from build123d import *

# Parameters (mm, degrees)
EXTRUDE_THIN1_DEPTH = 492.125
FILLET1_R           = 1.016


with BuildPart() as part:
    # Sketch1 → Extrude-Thin1 (new body)
    with BuildSketch(Plane.XY):
        with BuildLine():
            Line((0, 6.35), (0, 0))
            Line((0, 0), (-6.35, 0))
            Line((-6.35, 0), (-6.35, 3.96875))
            ThreePointArc((-6.35, 3.96875), (-14.128687, 6.629724), (-18.647706, 13.497563))
            ThreePointArc((-18.647706, 13.497563), (-20.900169, 25.701402), (-21.43125, 38.1))
            Line((-21.43125, 38.1), (-23.8125, 38.1))
            Line((-23.8125, 38.1), (-23.8125, 49.2125))
            Line((-23.8125, 49.2125), (-17.4625, 48.879711))
            Line((-17.4625, 48.879711), (-17.515673, 47.865103))
            Line((-17.515673, 47.865103), (-22.7965, 48.141859))
            Line((-22.7965, 48.141859), (-22.7965, 39.116))
            Line((-22.7965, 39.116), (-20.381189, 39.116))
            ThreePointArc((-20.381189, 39.116), (-19.947758, 26.334511), (-17.66389, 13.751258))
            ThreePointArc((-17.66389, 13.751258), (-13.09767, 7.130154), (-5.334, 5.029008))
            Line((-5.334, 5.029008), (-5.334, 1.016))
            Line((-5.334, 1.016), (-1.016, 1.016))
            Line((-1.016, 1.016), (-1.016, 6.35))
            Line((-1.016, 6.35), (0, 6.35))
        make_face()
    extrude(amount=-EXTRUDE_THIN1_DEPTH)

    # Fillet1
    fillet1_edges = [part.edges().sort_by_distance(p)[0] for p in [
        (-20.381189, 39.116, -246.0625),
        (-5.334, 5.029008, -246.0625),
        (0, 0, -246.0625),
        (-6.35, 0, -246.0625),
        (-23.8125, 38.1, -246.0625),
        (-23.8125, 49.2125, -246.0625),
    ]]
    fillet(fillet1_edges, radius=FILLET1_R)


solid = part.part
CAD build for the part. Positions are in the model's coordinates, mm. Coordinates: 2 decimals unless noted, no trailing zeros. Order: outer loops, then holes, each group sorted by start corner. A loop starts at its lowest first (then second) coordinate and runs counter-clockwise, first axis right, second up.
Item 1: Two-plate mould, pull along X, no slides. Class faces 1 (the face through (-20, 23, 0)), 2 (the face through (-20.88, 25.53, -242.62)), 3 (the face through (-19.91, 25.99, -242.62)), 4 (the face through (-13.59, 7.5, -242.62)): +X half, -X half, draft (parallel to the pull), parting line (faces both ways), or undercut.
Check sheet entries:
face 1: draft
face 2: -X half
face 3: +X half
face 4: undercut
Item 2: Band-saw the part on B-B on y = 19.5. List the corners of the cut face in (x, z) (3 decimals), plus the area to 3 significant figures.
Check sheet entries:
outline: (-19.976, -492.125) - (-18.943, -492.125) - (-18.943, 0) - (-19.976, 0) - close
area: 509 mm2
Item 3: Band-saw the part on A-A on z = -279.5. List the corners of the cut face in (x, y), plus the area to 3 significant figures.
Check sheet entries:
outline: (-23.81, 39.12) arc R1.02 ccw to (-22.8, 38.1) - (-21.43, 38.1) arc R88.9 ccw to (-18.65, 13.5) arc R12.7 ccw to (-6.35, 3.97) - (-6.35, 1.02) arc R1.02 ccw to (-5.33, 0) - (-1.02, 0) arc R1.02 ccw to (0, 1.02) - (0, 6.35) - (-1.02, 6.35) - (-1.02, 1.02) - (-5.33, 1.02) - (-5.33, 3.97) arc R1.02 ccw to (-6.35, 4.98) arc R11.68 cw to (-17.66, 13.75) arc R87.88 cw to (-20.42, 38.07) arc R1.02 ccw to (-21.43, 39.12) - (-22.8, 39.12) - (-22.8, 48.14) - (-17.52, 47.87) - (-17.46, 48.88) - (-22.74, 49.16) arc R1.02 ccw to (-23.81, 48.14) - close
area: 75.1 mm2
Item 4: Pin check, flat tips, straight feed: pin 1 Ø6 at (x, z) = (-9.5, -359) entering from -Y; pin 2 Ø8 at (x, z) = (-14, -234) entering from +Y; pin 3 Ø1.1 at (x, z) = (-22, -198) entering from +Y. Stop position of each tip, or through.
Check sheet entries:
pin 1: stops at y = 3.97
pin 2: stops at y = 48.91
pin 3: stops at y = 49.15
Item 5: Drill centre lines: L1, parallel to X at y = 3.5, z = -353.5; L2, parallel to Y at x = -7.5, z = -282; L3, parallel to Y at x = -3.25, z = -119.5. Where is each one in solid material? Low to high.
Check sheet entries:
L1: x = -6.35 to -5.33, -1.02 to 0
L2: y = 4.02 to 5.04
L3: y = 0 to 1.02
